from build123d import *

# Parameters (mm, degrees)
SKETCH1_R          = 85
BASE_FLANGE1_DEPTH = 3
SKETCH2_R          = 4.6
EXTRUDE1_DEPTH     = 3
SKETCH3_R          = 4.6
EXTRUDE2_DEPTH     = 3
CIRPATTERN1_COUNT  = 8
SKETCH4_R          = 2.1
CUT_EXTRUDE1_DEPTH = 10


# Sheet-metal steps are written as plain solids
with BuildPart() as part:
    # Sketch1 → Base-Flange1 (new body)
    with BuildSketch(Plane.XY):
        with BuildLine():
            Line((218, 218), (218, 275))
            Line((218, 275), (178, 275))
            Line((178, 275), (178, 245))
            ThreePointArc((178, 245), (0, 157.626305625), (-178, 245))
            Line((-178, 245), (-178, 275))
            Line((-178, 275), (-218, 275))
            Line((-218, 275), (-218, 218))
            Line((-218, 218), (-275, 218))
            Line((-275, 218), (-275, 178))
            Line((-275, 178), (-245, 178))
            ThreePointArc((-245, 178), (-157.626305625, 0), (-245, -178))
            Line((-245, -178), (-275, -178))
            Line((-275, -178), (-275, -218))
            Line((-275, -218), (-218, -218))
            Line((-218, -218), (-218, -275))
            Line((-218, -275), (-178, -275))
            Line((-178, -275), (-178, -245))
            ThreePointArc((-178, -245), (0, -157.626305625), (178, -245))
            Line((178, -245), (178, -275))
            Line((178, -275), (218, -275))
            Line((218, -275), (218, -218))
            Line((218, -218), (275, -218))
            Line((275, -218), (275, -178))
            Line((275, -178), (245, -178))
            ThreePointArc((245, -178), (157.626305625, 0), (245, 178))
            Line((245, 178), (275, 178))
            Line((275, 178), (275, 218))
            Line((275, 218), (218, 218))
        make_face()
        Circle(SKETCH1_R, mode=Mode.SUBTRACT)
    extrude(amount=BASE_FLANGE1_DEPTH)

    # Sketch2 → Extrude1 (cut)
    with BuildSketch(Plane.XY.offset(3)):
        with Locations((198, 262.5)):
            Circle(SKETCH2_R)
        with Locations((198, 232.5)):
            Circle(SKETCH2_R)
        with Locations((232.5, 198)):
            Circle(SKETCH2_R)
        with Locations((262.5, 198)):
            Circle(SKETCH2_R)
        with Locations(Location((262.5, -198, 0), (0, 0, 180))):
            Circle(SKETCH2_R)
        with Locations(Location((232.5, -198, 0), (0, 0, 180))):
            Circle(SKETCH2_R)
        with Locations(Location((198, -232.5, 0), (0, 0, 180))):
            Circle(SKETCH2_R)
        with Locations(Location((198, -262.5, 0), (0, 0, 180))):
            Circle(SKETCH2_R)
        with Locations((-198, -262.5)):
            Circle(SKETCH2_R)
        with Locations((-198, -232.5)):
            Circle(SKETCH2_R)
        with Locations((-232.5, -198)):
            Circle(SKETCH2_R)
        with Locations((-262.5, -198)):
            Circle(SKETCH2_R)
        with Locations(Location((-262.5, 198, 0), (0, 0, 180))):
            Circle(SKETCH2_R)
        with Locations(Location((-232.5, 198, 0), (0, 0, 180))):
            Circle(SKETCH2_R)
        with Locations(Location((-198, 232.5, 0), (0, 0, 180))):
            Circle(SKETCH2_R)
        with Locations(Location((-198, 262.5, 0), (0, 0, 180))):
            Circle(SKETCH2_R)
    extrude(amount=-EXTRUDE1_DEPTH, mode=Mode.SUBTRACT)

    # Sketch3 → Extrude2 (cut)
    with BuildSketch(Plane.XY.offset(3)):
        with Locations((0, 95)):
            Circle(SKETCH3_R)
    extrude2 = extrude(amount=-EXTRUDE2_DEPTH, mode=Mode.SUBTRACT)

    # CirPattern1: Extrude2 ×8 about axis
    cirpattern1_axis = Axis((0, 0, 0), (0, 0, 1))
    for i in range(1, CIRPATTERN1_COUNT):
        add(extrude2.rotate(cirpattern1_axis, i * 360 / CIRPATTERN1_COUNT), mode=Mode.SUBTRACT)

    # Sketch4 → Cut-Extrude1 (cut)
    with BuildSketch(Plane.XY.offset(3)):
        with Locations((-189.715728753, -189.715728753)):
            Circle(SKETCH4_R)
        with Locations((-171.330952442, -171.330952442)):
            Circle(SKETCH4_R)
        with Locations((-128.197438789, -128.197438789)):
            Circle(SKETCH4_R)
        with Locations((175.573593129, -175.573593129)):
            Circle(SKETCH4_R)
        with Locations((159.310137162, -159.310137162)):
            Circle(SKETCH4_R)
    extrude(amount=-CUT_EXTRUDE1_DEPTH, mode=Mode.SUBTRACT)


solid = part.part
Design review of the part built by this model. Coordinates are the model's own, in mm. Coordinates: 2 decimals unless noted, no trailing zeros. Order: outer loops, then holes, each group sorted by start corner. A loop starts at its lowest first (then second) coordinate and runs counter-clockwise, first axis right, second up. Notation, with made-up numbers: (40, -37) - (71, -37) arc R21 ccw to (71, -28) - close; hole circle Ø5 at (-26, -2). An arc over 180 degrees is marked (long way). Put each result on its own line as item: value.
1) The part is to be moulded in two halves that separate along Y. For faces 1 (the face through (-2.875, -157.645, 1.479)), 2 (the face through (-67.453, -51.721, 1.479)), 3 (the face through (2.875, 157.645, 1.479)), say which applies: released by +Y, released by -Y, zero draft, split by the parting line, or undercut.
Response values:
face 1: released by -Y
face 2: undercut
face 3: released by +Y
2) Insertion check: P1, Ø2, axis at x = 122.5, y = -55.5, coming from the -Z side; P2, Ø0.9, axis at x = -255, z = 1, coming from the +Y side; P3, Ø0.9, axis at y = 257, z = 2, coming from the +X side. Each pin has a flat end and moves straight along its axis. Give the tip position at first contact, or say it passes through.
Response values:
P1: stops at z = 0
P2: stops at y = 218
P3: stops at x = 218
3) Wall thickness on L1, parallel to X at y = -262.5, z = 0.8; L2, parallel to Y at x = 0, z = 0.7: over which ranges is each line inside the solid? List them lowest first. Write a range as from..to.
Response values:
L1: x = -218..-202.6, -193.4..-178, 178..193.4, 202.6..218
L2: y = -157.63..-99.6, -90.4..-85, 85..90.4, 99.6..157.63
4) Take a section at A-A, the plane x = 46. Give the boundary of the cut face in (y, z).
Response values:
outline: (-162.38, 0) - (-71.48, 0) - (-71.48, 3) - (-162.38, 3) - close; (71.48, 0) - (162.38, 0) - (162.38, 3) - (71.48, 3) - close
5) Take a section at C-C, the plane x = -44. Give the boundary of the cut face in (y, z).
Response values:
outline: (-161.97, 0) - (-72.73, 0) - (-72.73, 3) - (-161.97, 3) - close; (72.73, 0) - (161.97, 0) - (161.97, 3) - (72.73, 3) - close
6) Take a section at D-D, the plane z = 1.4. Count the separate pieces of the cut face and the enclosed holes in it, and give its area (3 significant figures).
Response values:
separate pieces: 1
enclosed holes: 30
area: 136,000 mm²
7) Take a section at B-B, the plane y = 133. Give the boundary of the cut face in (x, z).
Response values:
outline: (-201.14, 0) - (201.14, 0) - (201.14, 3) - (-201.14, 3) - close
